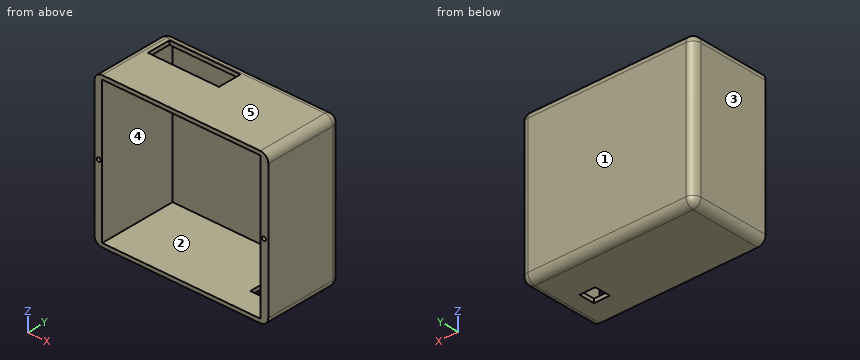
```python
from build123d import *

# Parameters (mm, degrees)
F0_W      = 110
F0_H      = 95
F1_DEPTH  = 50
F2_W      = 100
F2_H      = 90
F3_DEPTH  = 49
F4_R      = 1.25
F5_DEPTH  = 5
F6_R      = 5
F7_W      = 45
F7_H      = 15
F8_DEPTH  = 25
F9_W      = 10
F9_H      = 10
F10_DEPTH = 5


with BuildPart() as f1:
    # F0 (on Front) → F1 (new body)
    with BuildSketch(Plane.XZ):
        with Locations((-17.189732, -22.157951)):
            Rectangle(F0_W, F0_H)
    extrude(amount=F1_DEPTH)

    # F2 (on face) → F3 (cut)
    with BuildSketch(Plane.XZ.offset(50)):
        with Locations((-17.189732, -22.157951)):
            Rectangle(F2_W, F2_H)
    extrude(amount=-F3_DEPTH, mode=Mode.SUBTRACT)

    # F4 (on face) → F5 (cut)
    with BuildSketch(Plane.XZ.offset(50)):
        with Locations((-69.439732, -22.157951)):
            Circle(F4_R)
        with Locations((35.060268, -22.157951)):
            Circle(F4_R)
    extrude(amount=-F5_DEPTH, mode=Mode.SUBTRACT)

    # F6
    f6_edges = [f1.edges().sort_by_distance(p)[0] for p in [
        (-72.189732, -25, -69.657951),
        (-72.189732, -25, 25.342049),
        (37.810268, -25, -69.657951),
        (37.810268, -25, 25.342049),
        (37.810268, 0, -22.157951),
        (-72.189732, 0, -22.157951),
        (-17.189732, 0, -69.657951),
        (-17.189732, 0, 25.342049),
    ]]
    fillet(f6_edges, radius=F6_R)

    # F7 (on face) → F8 (cut)
    with BuildSketch(Plane.XY.offset(25.342049)):
        with Locations((-42.189732, -13.5)):
            Rectangle(F7_W, F7_H)
    extrude(amount=-F8_DEPTH, mode=Mode.SUBTRACT)

    # F9 (on face) → F10 (cut)
    with BuildSketch(Plane(origin=(0, 0, -69.657951), x_dir=(1, 0, 0), z_dir=(0, 0, -1))):
        with Locations((17.810268, 30)):
            Rectangle(F9_W, F9_H)
    extrude(amount=-F10_DEPTH, mode=Mode.SUBTRACT)


solid = f1.part
```
Input: part model. Units: mm. Frame: model coordinates. Face numbers are marked on the shaded views. A direction names the side the tool comes from. Round coordinates to 2 decimals unless told otherwise and drop trailing zeros. Write each loop counter-clockwise with the first axis right and the second up, starting at its lowest first coordinate (ties: lowest second). Pieces come first, ordered by that corner, then holes. Notation, with made-up numbers: (85.5, 29) -> (103.5, 29) arc R26 cw to (103.5, 48) -> close; hole circle Ø11 at (35.25, -22.75). An arc over 180 degrees is marked (long way). Answer as CSV lines item,"result".
1. Reachability of the marked faces 4 and 5 from +Z, -Z, +X, -X, +Y, -Y: full face, straight path, thin tool, end or side. Return the list, or none.
Geometry says:
face 4,"-Y"
face 5,"+Z, +X, -X, +Y, -Y"
2. Section D-D (x = 0.5). Return the cut outline in (y, z).
Geometry says:
outline,"(-50, -69.66) -> (-5, -69.66) arc R5 ccw to (0, -64.66) -> (0, 20.34) arc R5 ccw to (-5, 25.34) -> (-50, 25.34) -> (-50, 22.84) -> (-1, 22.84) -> (-1, -67.16) -> (-50, -67.16) -> close"
3. Section B-B (y = -39). Return the cut outline in (x, z), plus the area to 3 significant figures.
Geometry says:
outline,"(-72.19, -64.66) arc R5 ccw to (-67.19, -69.66) -> (32.81, -69.66) arc R5 ccw to (37.81, -64.66) -> (37.81, 20.34) arc R5 ccw to (32.81, 25.34) -> (-67.19, 25.34) arc R5 ccw to (-72.19, 20.34) -> close; hole (-67.19, -67.16) -> (32.81, -67.16) -> (32.81, 22.84) -> (-67.19, 22.84) -> close"
area,"1,430 mm^2"
4. Section A-A (x = 15.5). Return the cut outline in (y, z).
Geometry says:
outline,"(-50, -69.66) -> (-35, -69.66) -> (-35, -67.16) -> (-50, -67.16) -> close; (-50, 22.84) -> (-1, 22.84) -> (-1, -67.16) -> (-25, -67.16) -> (-25, -69.66) -> (-5, -69.66) arc R5 ccw to (0, -64.66) -> (0, 20.34) arc R5 ccw to (-5, 25.34) -> (-50, 25.34) -> close"
5. Contact query for flat-ended pins moving along their axis: P1, Ø2, axis at y = -31.5, z = -68.5, coming from the -X side; P2, Ø1.2, axis at x = -36, z = 24.5, coming from the +Y side; P3, Ø3, axis at y = -28.5, z = -68, coming from the +X side. Output: stop coordinate, or through.
Geometry says:
P1,"stops at x = -71.3"
P2,"stops at y = -1.49"
P3,"stops at x = 37.46"
6. Section C-C (z = -2.5). Return the cut outline in (x, y).
Geometry says:
outline,"(-72.19, -50) -> (-67.19, -50) -> (-67.19, -1) -> (32.81, -1) -> (32.81, -50) -> (37.81, -50) -> (37.81, -5) arc R5 ccw to (32.81, 0) -> (-67.19, 0) arc R5 ccw to (-72.19, -5) -> close"
7. Mould query, pull axis X, two halves, no side actions, for the marked faces 1, 2 and 3. Classes: +X half, -X half, draft (parallel to the pull), parting line (faces both ways), or undercut.
Geometry says:
face 1,"draft"
face 2,"undercut"
face 3,"-X half"
8. Ray query, L1, parallel to Z at x = -4, y = -43; L2, parallel to X at y = -35, z = -47.5; L3, parallel to Y at x = 13, z = -38.5. Return the intervals inside material, ascending. Write a range as [from, to].
Geometry says:
L1,"z = [-69.66, -67.16], [22.84, 25.34]"
L2,"x = [-72.19, -67.19], [32.81, 37.81]"
L3,"y = [-1, 0]"
